Drawing for the job (mm, zero at the part's lowest x, y, z). A direction names the side the tool comes from. Coordinates: 2 decimals unless noted, no trailing zeros. Write each loop counter-clockwise with the first axis right and the second up, starting at its lowest first coordinate (ties: lowest second). Pieces come first, ordered by that corner, then holes. Notation, with made-up numbers: M 50.5,60 L 82.5,60 A29 ccw 82.5,98 Z; hole C -35.75,73 d11. An arc over 180 degrees is marked long. Use a Markdown table: item, result. Add a question column.
Q1. Slice it at D-D on y = 21. Write the cut outline in (x, z), then the cut area to 3 significant figures.
Q2. Slice it at C-C on x = 61.5. Write the cut outline in (y, z), then the cut area to 4 significant figures.
Q3. Tool access for the marked faces 1, 2, 3 and 4: list every direction of +Z, -Z, +X, -X, +Y, -Y with a clear straight run to the whole face (end or side of a thin tool).
Q4. Mould opens along Y. For the marked faces 5, 6, 7 and 8 say: released by +Y, released by -Y, zero draft, split by the parting line, or undercut.
Q5. Pin check, flat tips, straight feed: pin 1 Ø8.5 at (y, z) = (20, 40) entering from +X; pin 2 Ø12.5 at (x, z) = (39.5, 14) entering from +Y; pin 3 Ø9 at (x, z) = (12, 21.5) entering from +Y. Stop position of each tip, or through.
Q6. Wall check: L1, parallel to Y at x = 12.5, z = 20.5; L2, parallel to Z at x = 7, y = 42.5; L3, parallel to Y at x = 6.5, z = 4. Give the ranges that are in metal, low to high. Write a range as from..to.
Q7. Slice it at B-B on z = 4. Write the cut outline in (x, y), then the cut area to 3 significant figures.
Q8. Slice it at A-A on y = 56. Write the cut outline in (x, z).
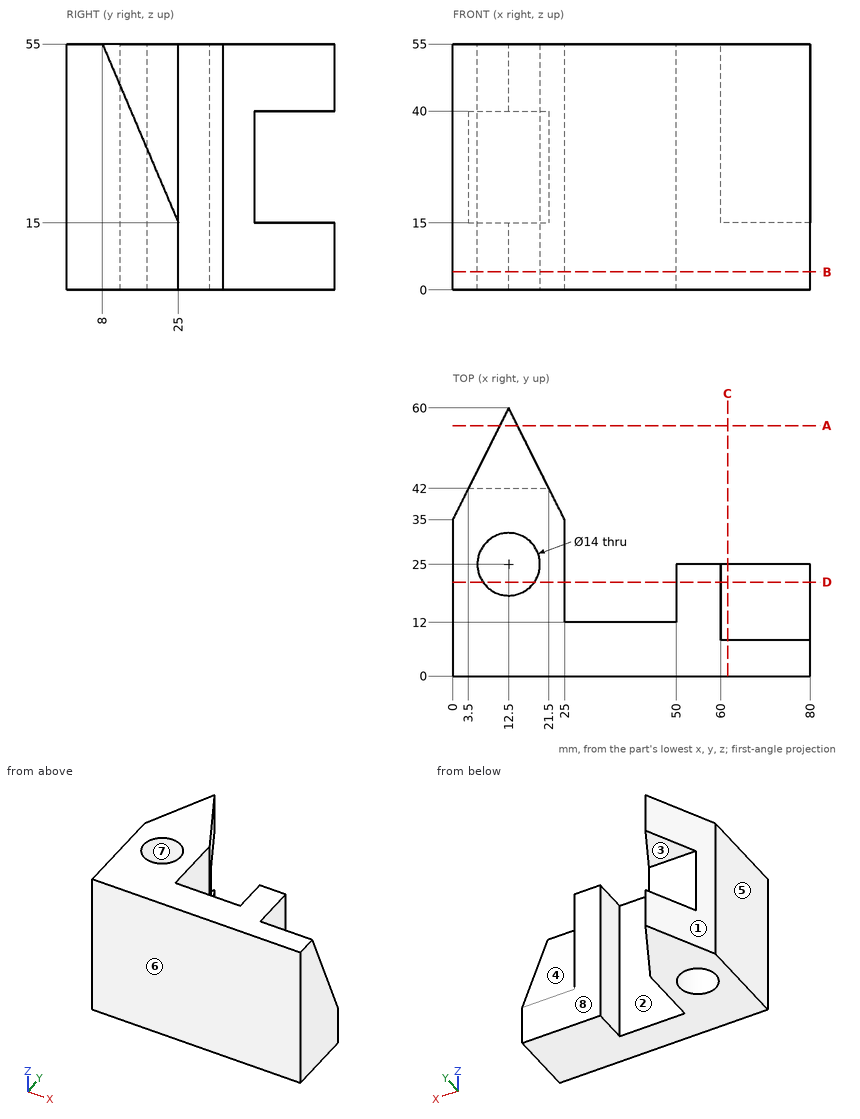
Recorded:
| question | item | result |
|---|---|---|
| 1 | outline | M 0,0 L 6.76,0 L 6.76,55 L 0,55 Z; M 18.24,0 L 25,0 L 25,55 L 18.24,55 Z; M 50,0 L 80,0 L 80,24.41 L 60,24.41 L 60,55 L 50,55 Z |
| 1 | area | 1,780 mm² |
| 2 | outline | M 0,0 L 25,0 L 25,15 L 8,55 L 0,55 Z |
| 2 | area | 1,035 mm² |
| 3 | face 1 | +Z, -Z, -X, +Y |
| 3 | face 2 | +Z, -Z, +Y |
| 3 | face 3 | +X, -X, +Y |
| 3 | face 4 | +Z, +X, +Y |
| 4 | face 5 | zero draft |
| 4 | face 6 | released by -Y |
| 4 | face 7 | undercut |
| 4 | face 8 | released by +Y |
| 5 | pin 1 | x = 60 |
| 5 | pin 2 | y = 12 |
| 5 | pin 3 | y = 42 |
| 6 | L1 | 0..18, 32..42 |
| 6 | L2 | 0..15, 40..55 |
| 6 | L3 | 0..21.39, 28.61..48 |
| 7 | outline | M 0,0 L 80,0 L 80,25 L 50,25 L 50,12 L 25,12 L 25,35 L 12.5,60 L 0,35 Z; hole C 12.5,25 d14 |
| 7 | area | 2,080 mm² |
| 8 | outline | M 10.5,0 L 14.5,0 L 14.5,15 L 10.5,15 Z; M 10.5,40 L 14.5,40 L 14.5,55 L 10.5,55 Z |
